from build123d import *

# Parameters (mm, degrees)
ESQUISSE1_W             = 100
ESQUISSE1_H             = 270
BOSS_EXTRU_1_DEPTH      = 5
ESQUISSE2_W             = 100
ESQUISSE2_H             = 270
ESQUISSE2_W_2           = 90
ESQUISSE2_H_2           = 260
BOSS_EXTRU_2_DEPTH      = 70
ESQUISSE3_W             = 65
ESQUISSE3_H             = 270
BOSS_EXTRU_4_DEPTH      = 5
ESQUISSE5_W             = 90
ESQUISSE5_H             = 5
ESQUISSE5_W_2           = 89.831851537
BOSS_EXTRU_5_DEPTH      = 5
ESQUISSE6_W             = 219.831851537
ESQUISSE6_H             = 270
ESQUISSE6_W_2           = 209.831851537
ESQUISSE6_H_2           = 260
BOSS_EXTRU_6_DEPTH      = 50
ESQUISSE7_R             = 10
ENL_V_MAT_EXTRU_1_DEPTH = 340.626590193
ESQUISSE8_W             = 159.831851537
ESQUISSE8_H             = 210
BOSS_EXTRU_7_DEPTH      = 5


with BuildPart() as part:
    # Esquisse1 → Boss.-Extru.1 (new body)
    with BuildSketch(Plane.XY):
        with Locations((-50, 135)):
            Rectangle(ESQUISSE1_W, ESQUISSE1_H)
    extrude(amount=BOSS_EXTRU_1_DEPTH)

    # Esquisse2 → Boss.-Extru.2 (add)
    with BuildSketch(Plane.XY.offset(5)):
        with Locations((-50, 135)):
            Rectangle(ESQUISSE2_W, ESQUISSE2_H)
        with Locations((-50, 135)):
            Rectangle(ESQUISSE2_W_2, ESQUISSE2_H_2, mode=Mode.SUBTRACT)
    extrude(amount=BOSS_EXTRU_2_DEPTH)

    # Esquisse3 → Boss.-Extru.4 (add)
    with BuildSketch(Plane.XY.offset(75)):
        with Locations((-127.5, 135)):
            Rectangle(ESQUISSE3_W, ESQUISSE3_H)
        with Locations((27.331851537, 135)):
            Rectangle(ESQUISSE3_W, ESQUISSE3_H)
    extrude(amount=BOSS_EXTRU_4_DEPTH)

    # Esquisse5 → Boss.-Extru.5 (add)
    with BuildSketch(Plane.XY.offset(75)):
        with Locations((-50, 267.5)):
            Rectangle(ESQUISSE5_W, ESQUISSE5_H)
        with Locations((-50.084074231, 2.5)):
            Rectangle(ESQUISSE5_W_2, ESQUISSE5_H)
    extrude(amount=BOSS_EXTRU_5_DEPTH)

    # Esquisse6 → Boss.-Extru.6 (add)
    with BuildSketch(Plane.XY.offset(80)):
        with Locations((-50.084074231, 135)):
            Rectangle(ESQUISSE6_W, ESQUISSE6_H)
        with Locations((-50.084074231, 135)):
            Rectangle(ESQUISSE6_W_2, ESQUISSE6_H_2, mode=Mode.SUBTRACT)
    extrude(amount=BOSS_EXTRU_6_DEPTH)

    # Esquisse7 → Enlèv. mat.-Extru.1 (cut, through all)
    with BuildSketch(Plane.ZY.offset(100)):
        with Locations((30, 140)):
            Circle(ESQUISSE7_R)
        with Locations((30, 38.975952284)):
            Circle(ESQUISSE7_R)
        with Locations((30, 236.400600349)):
            Circle(ESQUISSE7_R)
    extrude(amount=-ENL_V_MAT_EXTRU_1_DEPTH, mode=Mode.SUBTRACT)

    # Esquisse8 → Boss.-Extru.7 (add)
    with BuildSketch(Plane.XY.offset(130)):
        Polygon((-160, 270), (-130, 270), (59.831851537, 270), (59.831851537, 240), (59.831851537, 0), (29.831851537, 0), (-130, 0), (-160, 0), align=None)
        with Locations((-50.084074231, 135)):
            Rectangle(ESQUISSE8_W, ESQUISSE8_H, mode=Mode.SUBTRACT)
    extrude(amount=BOSS_EXTRU_7_DEPTH)


solid = part.part
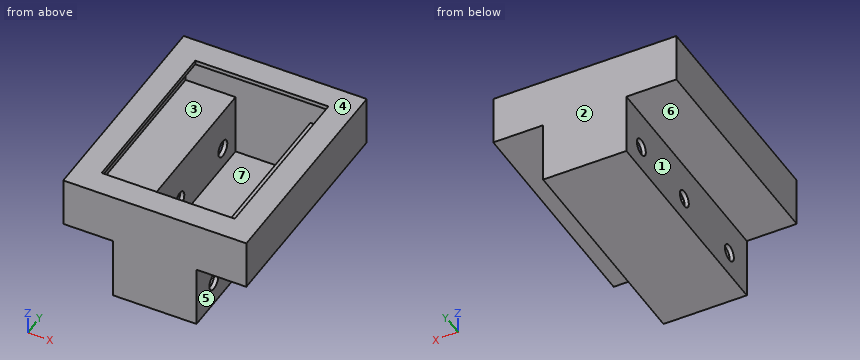
Build history of the part. All positions in model axes, mm. Face numbers are marked on the shaded views. A direction names the side the tool comes from. Give positions to 0.01 mm unless a question says otherwise; leave off trailing zeros. Order: outer loops, then holes, each group sorted by start corner. A loop starts at its lowest first (then second) coordinate and runs counter-clockwise, first axis right, second up. Notation, with made-up numbers: M -20.75,-38 L 32.25,-38 A22 ccw 32.25,1 Z; hole C -22,37 d10. An arc over 180 degrees is marked long. Put each result on its own line as item: value.
Item 1: Cut at A-A on y = 140. Count the separate pieces of the cut face and the enclosed holes in it, then the cut area to 3 significant figures.
Results are:
separate pieces: 3
enclosed holes: 0
area: 2,450 mm2
Item 2: Pull direction X, two halves, no side cores. Call the marked faces 1, 2 and 3: +X half, -X half, draft (parallel to the pull), parting line (faces both ways), or undercut.
Results are:
face 1: -X half
face 2: draft
face 3: undercut
Item 3: Drop flat-ended pins along their axis: pin 1 Ø18 at (y, z) = (236.4, 30) entering from +X; pin 2 Ø5 at (x, y) = (-42, 220) entering from +Z; pin 3 Ø22.5 at (y, z) = (195.5, 39.5) entering from +X; pin 4 Ø1 at (x, y) = (21.5, 121.5) entering from +Z. Give the stop position or say it passes through.
Results are:
pin 1: through
pin 2: z = 5
pin 3: x = 0
pin 4: z = 80
Item 4: Cut at C-C on z = 104. Write the cut outline in (x, y).
Results are:
outline: M -160,0 L 59.83,0 L 59.83,270 L -160,270 Z; hole M -155,5 L 54.83,5 L 54.83,265 L -155,265 Z
Item 5: Wall check: probe 1 along Y at (x, z) = (-1.65, 30); probe 2 along X at (y, z) = (176.5, 90); probe 3 along Z at (x, y) = (-138, 187.5). Give the ranges that are in metal, low to high.
Results are:
probe 1: 0 to 28.98, 48.98 to 130, 150 to 226.4, 246.4 to 270
probe 2: -160 to -155, 54.83 to 59.83
probe 3: 75 to 80, 130 to 135
Item 6: Cut at D-D on x = -55. Write the cut outline in (y, z).
Results are:
outline: M 0,0 L 270,0 L 270,135 L 240,135 L 240,130 L 265,130 L 265,5 L 5,5 L 5,130 L 30,130 L 30,135 L 0,135 Z
Item 7: Which spindle directions (+Z, -Z, +X, -X, +Y, -Y) get a long thin tool onto all of the face, cutting with end or side? Do the marked faces 4, 5, 6 and 7. Say none if no direction does.
Results are:
face 4: +Z, +X, -X, +Y, -Y
face 5: -Z, +X, +Y, -Y
face 6: -Z, -X, +Y, -Y
face 7: none
